```python
from build123d import *

# Parameters (mm, degrees)
SKETCH1_R           = 3.1
BOSS_EXTRUDE1_DEPTH = 3
FILLET1_R           = 3
FILLET2_R           = 1


with BuildPart() as part:
    # Sketch1 → Boss-Extrude1 (new body)
    with BuildSketch(Plane(origin=(0, 0, 0), x_dir=(1, 0, 0), z_dir=(0, 1, 0))):
        with BuildLine():
            ThreePointArc((21.667324002, 49.462380357), (-38.183766184, -38.183766184), (49.462380357, 21.667324002))
            ThreePointArc((49.462380357, 21.667324002), (46.165505457, 19.845504593), (42.585510083, 18.674162122))
            ThreePointArc((42.585510083, 18.674162122), (32.880465325, 32.880465325), (18.674162122, 42.585510083))
            ThreePointArc((18.674162122, 42.585510083), (19.845504593, 46.165505457), (21.667324002, 49.462380357))
        make_face()
        with Locations(Location((10, 0, 0), (0, 0, 270))):
            Circle(SKETCH1_R, mode=Mode.SUBTRACT)
        with Locations(Location((0, 20, 0), (0, 0, 270))):
            Circle(SKETCH1_R, mode=Mode.SUBTRACT)
        with Locations(Location((0, -20, 0), (0, 0, 270))):
            Circle(SKETCH1_R, mode=Mode.SUBTRACT)
        with Locations(Location((-10, 0, 0), (0, 0, 270))):
            Circle(SKETCH1_R, mode=Mode.SUBTRACT)
    extrude(amount=BOSS_EXTRUDE1_DEPTH)

    # Fillet1
    fillet1_edges = [part.edges().sort_by_distance(p)[0] for p in [
        (49.462380357, 1.5, -21.667324002),
        (21.667324002, 1.5, -49.462380357),
    ]]
    fillet(fillet1_edges, radius=FILLET1_R)

    # Fillet2
    fillet2_edges = [part.edges().sort_by_distance(p)[0] for p in [
        (18.674162122, 1.5, -42.585510083),
        (42.585510083, 1.5, -18.674162122),
    ]]
    fillet(fillet2_edges, radius=FILLET2_R)


solid = part.part
```
CAD build for the part. Positions are in the model's coordinates, mm. A direction names the side the tool comes from. Give positions to 0.01 mm unless a question says otherwise; leave off trailing zeros. Write each loop counter-clockwise with the first axis right and the second up, starting at its lowest first coordinate (ties: lowest second). Pieces come first, ordered by that corner, then holes. Notation, with made-up numbers: (43, 24) -> (73, 24) arc R22 cw to (73, 39) -> close; hole circle Ø11 at (15.25, 54). An arc over 180 degrees is marked (long way). Write each question's results on one line, items separated by ' | '.
1. Cut at A-A, the plane z = 0. Write the cut outline in (x, y), then the cut area to 3 significant figures.
Geometry check:
outline: (-54, 0) -> (-13.1, 0) -> (-13.1, 3) -> (-54, 3) -> close; (-6.9, 0) -> (6.9, 0) -> (6.9, 3) -> (-6.9, 3) -> close; (13.1, 0) -> (54, 0) -> (54, 3) -> (13.1, 3) -> close | area: 287 mm²
2. Cut at C-C, the plane y = 1.2. Give the number of separate pieces and of enclosed holes in the cut face, then the cut area to 3 significant figures.
Geometry check:
separate pieces: 1 | enclosed holes: 4 | area: 8,750 mm²
3. Wall check: probe 1 along X at (y, z) = (1.9, 0); probe 2 along X at (y, z) = (1.85, -20); probe 3 along X at (y, z) = (0.2, 21.5). Give the ranges that are in metal, low to high. Write a range as [from, to].
Geometry check:
probe 1: [-54, -13.1], [-6.9, 6.9], [13.1, 54] | probe 2: [-50.16, -3.1], [3.1, 41.98], [46.51, 49.38] | probe 3: [-49.54, -2.71], [2.71, 49.54]
4. Which spindle directions (+Z, -Z, +X, -X, +Y, -Y) get a long thin tool onto all of the face, cutting with end or side? Do faces 4 (the flat face through (-1, 0, -1)), 5 (the cylindrical face through (45.097, 1.479, -19.417)). Say none if no direction does.
Geometry check:
face 4: +Z, -Z, +X, -X, -Y | face 5: -Z, +Y, -Y
5. Cut at B-B, the plane x = 0. Write the cut outline in (y, z), then the cut area to 3 significant figures.
Geometry check:
outline: (0, -54) -> (3, -54) -> (3, -23.1) -> (0, -23.1) -> close; (0, -16.9) -> (3, -16.9) -> (3, 16.9) -> (0, 16.9) -> close; (0, 23.1) -> (3, 23.1) -> (3, 54) -> (0, 54) -> close | area: 287 mm²
6. Two-plate mould, pull along X, no slides. Class faces 1 (the flat face through (-1, 3, -1)), 2 (the cylindrical face through (19.4, 1.48, -45.05)), 3 (the cylindrical face through (-1.886, 1.479, 17.54)): pulls with the +X half, pulls with the -X half, needs draft (parallel to the pull), parting line crosses it, or undercut.
Geometry check:
face 1: needs draft | face 2: pulls with the +X half | face 3: undercut
7. Cut at D-D, the plane x = -39. Write the cut outline in (y, z), then the cut area to 3 significant figures.
Geometry check:
outline: (0, -37.35) -> (3, -37.35) -> (3, 37.35) -> (0, 37.35) -> close | area: 224 mm²
8. Drop flat-ended pins along their axis: P1, Ø1, axis at x = -32.5, y = 0.5, coming from the +Z side; P2, Ø1, axis at x = 8.5, y = 1, coming from the +Z side; P3, Ø1.5, axis at y = 2.5, z = -18, coming from the +X side. Give the stop position or say it passes through.
Geometry check:
P1: z = 43.5 | P2: z = 53.4 | P3: x = 51.17
